Build history of the part. All positions in model axes, mm. A direction names the side the tool comes from. Coordinates: 2 decimals unless noted, no trailing zeros. Order: outer loops, then holes, each group sorted by start corner. A loop starts at its lowest first (then second) coordinate and runs counter-clockwise, first axis right, second up. Notation, with made-up numbers: M 76,37.25 L 111,37.25 A9 ccw 111,50.25 Z; hole C -22.5,89 d10. An arc over 180 degrees is marked long. Write item = value, one per line. Start each with the question number.
Q1. Drill centre lines: probe 1 along X at (y, z) = (1.2, 0) (3 decimals); probe 2 along Y at (x, z) = (-22.5, 3.25); probe 3 along Y at (x, z) = (-4.5, -2). Where is each one in solid material? Low to high.
Q2. Pin check, flat tips, straight feed: P1, Ø4, axis at x = -24, z = -2, coming from the +Y side; P2, Ø3, axis at x = -23, z = -4.5, coming from the -Y side; P3, Ø7, axis at x = -13, z = 1, coming from the +Y side; P4, Ø1.3, axis at x = -7, y = 1, coming from the +Z side (3 decimals). Stop position of each tip, or through.
Q3. 3-axis set-ups, long thin cutter, end or side, ignore diameter. For faces 1 (the face through (-23.1, 3.302, -1.4)), 2 (the face through (-13, 1, 3.175)), 3 (the face through (-29, 2.54, 0)), 4 (the face through (1.285, 5.671, 0.819)): which of +Z, -Z, +X, -X, +Y, -Y reach the whole face in a straight line?
Q4. Pull direction X, two halves, no side cores. Call faces 5 (the face through (-12, 0, 0)), 6 (the face through (-27.653, 1.674, 1.172)), 7 (the face through (-8, 2.54, 0)), 8 (the face through (-28.574, 1.252, 0.07)): released by +X, released by -X, zero draft, split by the parting line, or undercut.
Q5. Band-saw the part on D-D on x = -15.5. Write the cut outline in (y, z) (3 decimals).
Q6. Band-saw the part on A-A on z = 0. Write the cut outline in (x, y) (3 decimals).
Q7. Band-saw the part on B-B on y = 2. Write the cut outline in (x, z) (3 decimals), plus the area to 3 significant figures.
Q8. Band-saw the part on C-C on y = 5.25. Write the cut outline in (x, z), plus the area to 3 significant figures.
```python
from build123d import *

# Parameters (mm, degrees)
BOSS_EXTRUDE1_DEPTH = 2.54
SKETCH2_R           = 1.524
BOSS_EXTRUDE2_DEPTH = 6.35
SKETCH3_R           = 2.54
CUT_EXTRUDE1_DEPTH  = 30.443738723
BOSS_EXTRUDE3_START = 0.762
SKETCH4_R           = 6.35
SKETCH4_R_2         = 2.54
BOSS_EXTRUDE3_DEPTH = 0.762


with BuildPart() as part:
    # Sketch1 → Boss-Extrude1 (new body)
    with BuildSketch(Plane(origin=(0, 0, 0), x_dir=(1, 0, 0), z_dir=(0, 1, 0))):
        with BuildLine():
            Line((0, -3.175), (-25.4, -3.175))
            ThreePointArc((-25.4, -3.175), (-28.575, 0), (-25.4, 3.175))
            Line((-25.4, 3.175), (0, 3.175))
            ThreePointArc((0, 3.175), (3.175, 0), (0, -3.175))
        make_face()
    extrude(amount=BOSS_EXTRUDE1_DEPTH)

    # Sketch2 → Boss-Extrude2 (add)
    with BuildSketch(Plane(origin=(0, 2.54, 0), x_dir=(1, 0, 0), z_dir=(0, 1, 0))):
        with Locations(Location((0, 0, 0), (0, 0, 270))):
            Circle(SKETCH2_R)
    extrude(amount=BOSS_EXTRUDE2_DEPTH)

    # Sketch3 → Cut-Extrude1 (cut, through all)
    with BuildSketch(Plane(origin=(0, 2.54, 0), x_dir=(1, 0, 0), z_dir=(0, 1, 0))):
        with Locations(Location((-25.4, 0, 0), (0, 0, 270))):
            Circle(SKETCH3_R)
    extrude(amount=-CUT_EXTRUDE1_DEPTH, mode=Mode.SUBTRACT)

    # Sketch4 → Boss-Extrude3 (add)
    with BuildSketch(Plane(origin=(0, 2.54, 0), x_dir=(1, 0, 0), z_dir=(0, 1, 0)).offset(BOSS_EXTRUDE3_START)):
        with Locations(Location((-25.4, 0, 0), (0, 0, 30))):
            Circle(SKETCH4_R)
        with Locations(Location((-25.4, 0, 0), (0, 0, 270))):
            Circle(SKETCH4_R_2, mode=Mode.SUBTRACT)
    extrude(amount=-BOSS_EXTRUDE3_DEPTH)


solid = part.part
```
Recorded:
q1.probe_1 = -28.575 to -27.94, -22.86 to 3.175
q1.probe_2 = 2.54 to 3.3
q1.probe_3 = 0 to 2.54
q2.P1 = 3.3
q2.P2 = 0
q2.P3 = 2.54
q2.P4 = 3.175
q3.face_1 = +Z, -Z, -X, +Y
q3.face_2 = +Z, +X, -X, -Y
q3.face_3 = -X, -Y
q3.face_4 = +Y
q4.face_5 = zero draft
q4.face_6 = undercut
q4.face_7 = undercut
q4.face_8 = released by -X
q5.outline = M 0,-3.175 L 2.54,-3.175 L 2.54,3.175 L 0,3.175 Z
q6.outline = M -31.75,2.54 L -28.575,2.54 L -28.575,0 L -27.94,0 L -27.94,3.302 L -31.75,3.302 Z; M -22.86,0 L 3.175,0 L 3.175,2.54 L 1.524,2.54 L 1.524,8.89 L -1.524,8.89 L -1.524,2.54 L -19.05,2.54 L -19.05,3.302 L -22.86,3.302 Z
q7.outline = M -25.4,-3.175 L 0,-3.175 A3.175 ccw 0,3.175 L -25.4,3.175 A3.175 ccw Z; hole C -25.4,0 d5.08
q7.area = 173 mm2
q8.outline = C 0,0 d3.05
q8.area = 7.30 mm2
